from build123d import *

# Parameters (mm, degrees)
F1_DEPTH = 6.35
F2_R     = 3.175
F3_DEPTH = 1.27
F5_DEPTH = 12.7


with BuildPart() as f1:
    # F0 (on Front) → F1 (new body, symmetric)
    with BuildSketch(Plane.XZ):
        Polygon((-25.4, 25.4), (0, 0), (0, 25.4), align=None)
    extrude(amount=F1_DEPTH, both=True)

    # F2 (on face) → F3 (cut)
    with BuildSketch(Plane(origin=(0, 0, 0), x_dir=(0.7071067812, 0, -0.7071067812), z_dir=(-0.7071067812, 0, -0.7071067812))):
        with Locations((-13.97, 0)):
            Circle(F2_R)
        with Locations((-6.35, 0)):
            Circle(F2_R)
    extrude(amount=-F3_DEPTH, mode=Mode.SUBTRACT)

    # F4 (on face) → F5 (cut)
    with BuildSketch(Plane.XZ.offset(6.35)):
        Polygon((-25.4, 25.4), (-13.97, 13.97), (0, 13.97), (0, 25.4), align=None)
    extrude(amount=-F5_DEPTH, mode=Mode.SUBTRACT)


solid = f1.part
Check sheet for the modelled part. Datum: model origin and axes. Units: mm. A direction names the side the tool comes from. Coordinates: 2 decimals unless noted, no trailing zeros. Write each loop counter-clockwise with the first axis right and the second up, starting at its lowest first coordinate (ties: lowest second). Pieces come first, ordered by that corner, then holes.
Item 1: Mould release check, pull along Z, two halves, no side actions. Record for faces 1 (the face through (-3.011, 2.817, 3.897)), 2 (the face through (0, 0, 7)), 3 (the face through (-11.22, 1.93, 12.1)), 4 (the face through (-7, 0, 13.97)): released by +Z, released by -Z, zero draft, split by the parting line, or undercut.
Numbers:
face 1: undercut
face 2: zero draft
face 3: undercut
face 4: released by +Z
Item 2: Cross-section at A-A on y = 2.25. Record the boundary of the cut face in (x, z).
Numbers:
outline: (-13.97, 13.97) - (-11.46, 11.46) - (-10.56, 12.36) - (-7.4, 9.19) - (-8.29, 8.29) - (-6.07, 6.07) - (-5.18, 6.97) - (-2.01, 3.8) - (-2.91, 2.91) - (0, 0) - (0, 13.97) - close
Item 3: Cross-section at B-B on x = -0.75. Record the boundary of the cut face in (y, z).
Numbers:
outline: (-6.35, 0.75) - (6.35, 0.75) - (6.35, 13.97) - (-6.35, 13.97) - close
Item 4: Scan lines: probe 1 along X at (y, z) = (1.75, 12); probe 2 along Y at (x, z) = (-2.5, 4); probe 3 along X at (y, z) = (5.25, 1). Record each from-to range of solid material in increasing order.
Numbers:
probe 1: x = -12 to -11.5, -10.2 to 0
probe 2: y = -6.35 to -2.65, 2.65 to 6.35
probe 3: x = -1 to 0
Item 5: Access from +Z, -Z, +X, -X, +Y, -Y to the whole of each face (thin tool, end or side, straight path). Record for faces 5 (the face through (-7, 0, 7)), 6 (the face through (-9.012, -0.044, 10.808)).
Numbers:
face 5: -Z, -X, +Y, -Y
face 6: none
Item 6: Cross-section at C-C on z = 2. Record the boundary of the cut face in (x, y), then the cut area to 3 significant figures.
Numbers:
outline: (-2, -6.35) - (0, -6.35) - (0, 6.35) - (-2, 6.35) - close
area: 25.4 mm2
Item 7: Depth check by flat-ended pin: pin 1 Ø1.5 at (y, z) = (2.5, 2.5) entering from -X; pin 2 Ø1.5 at (x, y) = (-7, 0.5) entering from -Z; pin 3 Ø2 at (y, z) = (-3, 9) entering from -X. Enter the tip coordinate at first touch or a pass-through.
Numbers:
pin 1: stops at x = -3.24
pin 2: stops at z = 6.59
pin 3: stops at x = -9.99
Item 8: Cross-section at D-D on y = -0.75. Record the boundary of the cut face in (x, z), then the cut area to 3 significant figures.
Numbers:
outline: (-13.97, 13.97) - (-12.06, 12.06) - (-11.16, 12.96) - (-6.8, 8.59) - (-7.7, 7.7) - (-6.67, 6.67) - (-5.77, 7.57) - (-1.41, 3.21) - (-2.31, 2.31) - (0, 0) - (0, 13.97) - close
area: 81.9 mm2
